```python
from build123d import *

# Parameters (mm, degrees)
SKETCH1_R           = 2
BOSS_EXTRUDE1_DEPTH = 15
BOSS_EXTRUDE2_DEPTH = 15


with BuildPart() as part:
    # Sketch1 → Boss-Extrude1 (new body)
    with BuildSketch(Plane(origin=(0, 0, 0), x_dir=(0, 0, -1), z_dir=(1, 0, 0))):
        Circle(SKETCH1_R)
    extrude(amount=BOSS_EXTRUDE1_DEPTH)

    # Sketch2 → Boss-Extrude2 (add, through all)
    with BuildSketch(Plane(origin=(15, 0, 0), x_dir=(0, 0, -1), z_dir=(1, 0, 0))):
        Polygon((2.309401077, 0), (1.154700538, 2), (-1.154700538, 2), (-2.309401077, 0), (-1.154700538, -2), (1.154700538, -2), align=None)
    extrude(amount=-BOSS_EXTRUDE2_DEPTH)


solid = part.part
```
Part model, mm, in its own coordinate system. Coordinates: 2 decimals unless noted, no trailing zeros. Write each loop counter-clockwise with the first axis right and the second up, starting at its lowest first coordinate (ties: lowest second). Pieces come first, ordered by that corner, then holes.
Item 1: Slice it at A-A (x = 8.75). Write the cut outline in (y, z).
Item 2: Probe line 1 (Z direction, x = 11.75, y = -1.3); line 2 (Z direction, x = 10, y = 0.35); line 3 (Y direction, x = 3.75, z = -1.65). List the from-to ranges inside material, lowest first.
Item 3: Slice it at B-B (y = 1.7). Write the cut outline in (x, z), and give its area (3 significant figures).
Item 4: Slice it at C-C (z = 1.5). Write the cut outline in (x, y), and give its area (3 significant figures).
Results found:
1. outline: (-2, -1.15) - (0, -2.31) - (2, -1.15) - (2, 1.15) - (0, 2.31) - (-2, 1.15) - close
2. line 1: z = -1.56 to 1.56
2. line 2: z = -2.11 to 2.11
2. line 3: y = -1.14 to 1.14
3. outline: (0, -1.33) - (15, -1.33) - (15, 1.33) - (0, 1.33) - close
3. area: 39.8 mm2
4. outline: (0, -1.4) - (15, -1.4) - (15, 1.4) - (0, 1.4) - close
4. area: 42.1 mm2
